from build123d import *

# Parameters (mm, degrees)
FILLET1_R                            = 1.5
F_5_16_18_MAKE_SURE_TO_CHANGE_THIS_D = 7
CUT_EXTRUDE1_DEPTH                   = 42.853733412


with BuildPart() as part:
    # Sketch1 → Revolve1 (revolve)
    with BuildSketch(Plane.XY, mode=Mode.PRIVATE) as revolve1_sk:
        Polygon((0, 0), (38.1, 0), (38.1, 6.299999973), (4.7625, 6.299999973), (4.7625, 12.250000011), (0, 12.250000011), align=None)
    revolve(revolve1_sk.sketch.rotate(Axis((0, 0, 0), (-1, 0, 0)), 90), axis=Axis((0, 0, 0), (-1, 0, 0)))

    # Fillet1
    fillet1_edges = [part.edges().sort_by_distance(p)[0] for p in [
        (4.7625, 0, 6.299999973),
    ]]
    fillet(fillet1_edges, radius=FILLET1_R)

    # 5/16-18 MAKE SURE TO CHANGE THIS (through all)
    with Locations(Plane(origin=(38.1, 0, 0), x_dir=(0, 0, -1), z_dir=(1, 0, 0))):
        with Locations((0, 0)):
            Hole(F_5_16_18_MAKE_SURE_TO_CHANGE_THIS_D / 2)

    # Sketch4 → Cut-Extrude1 (cut, through all)
    with BuildSketch(Plane.ZY):
        with BuildLine():
            Line((-6.35, 10.475686148), (6.35, 10.475686148))
            ThreePointArc((6.35, 10.475686148), (0, 12.250000011), (-6.35, 10.475686148))
        make_face()
        with BuildLine():
            Line((6.35, -10.475686148), (-6.35, -10.475686148))
            ThreePointArc((-6.35, -10.475686148), (0, -12.250000011), (6.35, -10.475686148))
        make_face()
    extrude(amount=-CUT_EXTRUDE1_DEPTH, mode=Mode.SUBTRACT)


solid = part.part
Verification items for the finished model (mm, model axes). A direction names the side the tool comes from. Round coordinates to 2 decimals unless told otherwise and drop trailing zeros. Order: outer loops, then holes, each group sorted by start corner. A loop starts at its lowest first (then second) coordinate and runs counter-clockwise, first axis right, second up.
1. Section check A-A on y = 0. Record the cut outline in (x, z), then the cut area to 3 significant figures.
Final values:
outline: (0, -12.25) - (4.76, -12.25) - (4.76, -7.8) arc R1.5 cw to (6.26, -6.3) - (38.1, -6.3) - (38.1, -3.5) - (0, -3.5) - close; (0, 3.5) - (38.1, 3.5) - (38.1, 6.3) - (6.26, 6.3) arc R1.5 cw to (4.76, 7.8) - (4.76, 12.25) - (0, 12.25) - close
area: 271 mm2
2. Section check B-B on z = 0. Record the cut outline in (x, y), then the cut area to 3 significant figures.
Final values:
outline: (0, -10.48) - (4.76, -10.48) - (4.76, -7.8) arc R1.5 cw to (6.26, -6.3) - (38.1, -6.3) - (38.1, -3.5) - (0, -3.5) - close; (0, 3.5) - (38.1, 3.5) - (38.1, 6.3) - (6.26, 6.3) arc R1.5 cw to (4.76, 7.8) - (4.76, 10.48) - (0, 10.48) - close
area: 254 mm2
3. Thickness scan on L1, parallel to Y at x = 24, z = 0; L2, parallel to X at y = -4, z = -10.5; L3, parallel to Z at x = 25.5, y = 0.75. Record the ranges inside material, lowest first.
Final values:
L1: y = -6.3 to -3.5, 3.5 to 6.3
L2: x = 0 to 4.76
L3: z = -6.26 to -3.42, 3.42 to 6.26
4. Go/stop test with flat-tipped pins: P1, Ø6, axis at x = 26, y = 5, coming from the +Z side; P2, Ø10, axis at x = 28.5, y = 5.5, coming from the -Z side; P3, Ø2, axis at x = 7.5, y = -4.5, coming from the -Z side; P4, Ø4, axis at y = 3.5, z = 4.5, coming from the -X side. Record where each tip stops, or that it passes through.
Final values:
P1: stops at z = 5.97
P2: stops at z = -6.28
P3: stops at z = -5.24
P4: stops at x = 0
5. Release check for a two-part mould opening along Y. For faces 1 (the cylindrical face through (18.783, -1.341, 3.233)), 2 (the flat face through (2, -10.476, 0)), 3 (the cylindrical face through (2.35, 0.18, -12.25)) record: +Y half, -Y half, draft (parallel to the pull), parting line (faces both ways), or undercut.
Final values:
face 1: undercut
face 2: -Y half
face 3: parting line
6. Section check D-D on y = 9.25. Record the cut outline in (x, z), then the cut area to 3 significant figures.
Final values:
outline: (0, -8.03) - (4.76, -8.03) - (4.76, 8.03) - (0, 8.03) - close
area: 76.5 mm2
7. Access from +Z, -Z, +X, -X, +Y, -Y to the whole of each face (thin tool, end or side, straight path). Record for faces 4 (the flat face through (38.1, 3, 3)), 5 (the flat face through (4.762, 0, 8)).
Final values:
face 4: +Z, -Z, +X, +Y, -Y
face 5: +X
8. Section check C-C on x = 22. Record the cut outline in (y, z), then the cut area to 3 significant figures.
Final values:
outline: circle Ø12.6 at (0, 0); hole circle Ø7 at (0, 0)
area: 86.2 mm2
